For this review, take the finished solid that the model builds, in its own axes (mm). Round coordinates to 2 decimals unless told otherwise and drop trailing zeros. Order: outer loops, then holes, each group sorted by start corner. A loop starts at its lowest first (then second) coordinate and runs counter-clockwise, first axis right, second up.
```python
from build123d import *

# Parameters (mm, degrees)
F0_W     = 260.35
F0_H     = 25
F1_DEPTH = 7
F2_R     = 3.302
F3_DEPTH = 7
F4_W     = 30
F4_H     = 7
F5_DEPTH = 7


with BuildPart() as f1:
    # F0 (on Top) → F1 (new body)
    with BuildSketch(Plane.XY):
        Rectangle(F0_W, F0_H)
    extrude(amount=F1_DEPTH)

    # F2 (on face) → F3 (cut, through all)
    with BuildSketch(Plane.XY.offset(7)):
        with Locations((-120.175, 0)):
            Circle(F2_R)
        Circle(F2_R)
        with Locations((120.175, 0)):
            Circle(F2_R)
    extrude(amount=-F3_DEPTH, mode=Mode.SUBTRACT)

    # F4 (on face) → F5 (join)
    with BuildSketch(Plane(origin=(0, 12.5, 0), x_dir=(-1, 0, 0), z_dir=(0, 1, 0))):
        with Locations((100.175, 3.5)):
            Rectangle(F4_W, F4_H)
        with Locations((50.175, 3.5)):
            Rectangle(F4_W, F4_H)
        with Locations((-50.175, 3.5)):
            Rectangle(F4_W, F4_H)
        with Locations((-100.175, 3.5)):
            Rectangle(F4_W, F4_H)
    extrude(amount=F5_DEPTH)


solid = f1.part
```
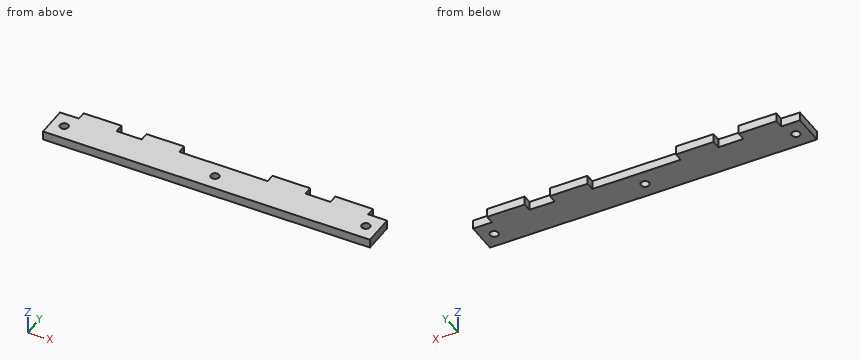
Q1. Take a section at B-B, the plane x = 0. State the section outline as (y, z) points.
Q2. Clearance check with flat-ended pins moving along their axes: pin 1 (3.5 mm diameter, centred on y = 16.5, z = 2.5, fed in from +X) (3 decimals); pin 2 (2 mm diameter, centred on x = -76.5, z = 2.5, fed in from +Y); pin 3 (2 mm diameter, centred on y = 14.5, z = 4.5, fed in from -X) (3 decimals). State where each tip first meets the part, or that it passes through.
Q3. Take a section at D-D, the plane y = 0. State the section outline as (x, z) points (3 decimals), plus the area to 3 significant figures.
Q4. Take a section at A-A, the plane y = 17. State the section outline as (x, z) points (3 decimals).
Q5. Wall thickness on line 1 (X direction, y = 13, z = 4.25) (3 decimals); line 2 (X direction, y = -1, z = 4) (3 decimals); line 3 (Y direction, x = -84, z = 4.5): over which ranges is each line inside the solid? List them lowest first.
Q6. Take a section at C-C, the plane z = 1.25. State the section outline as (x, y) points (3 decimals).
Working result:
1. outline: (-12.5, 0) - (-3.3, 0) - (-3.3, 7) - (-12.5, 7) - close; (3.3, 0) - (12.5, 0) - (12.5, 7) - (3.3, 7) - close
2. pin 1: stops at x = 115.175
2. pin 2: stops at y = 12.5
2. pin 3: stops at x = -115.175
3. outline: (-130.175, 0) - (-123.477, 0) - (-123.477, 7) - (-130.175, 7) - close; (-116.873, 0) - (-3.302, 0) - (-3.302, 7) - (-116.873, 7) - close; (3.302, 0) - (116.873, 0) - (116.873, 7) - (3.302, 7) - close; (123.477, 0) - (130.175, 0) - (130.175, 7) - (123.477, 7) - close
3. area: 1,680 mm2
4. outline: (-115.175, 0) - (-85.175, 0) - (-85.175, 7) - (-115.175, 7) - close; (-65.175, 0) - (-35.175, 0) - (-35.175, 7) - (-65.175, 7) - close; (35.175, 0) - (65.175, 0) - (65.175, 7) - (35.175, 7) - close; (85.175, 0) - (115.175, 0) - (115.175, 7) - (85.175, 7) - close
5. line 1: x = -115.175 to -85.175, -65.175 to -35.175, 35.175 to 65.175, 85.175 to 115.175
5. line 2: x = -130.175 to -123.322, -117.028 to -3.147, 3.147 to 117.028, 123.322 to 130.175
5. line 3: y = -12.5 to 12.5
6. outline: (-130.175, -12.5) - (130.175, -12.5) - (130.175, 12.5) - (115.175, 12.5) - (115.175, 19.5) - (85.175, 19.5) - (85.175, 12.5) - (65.175, 12.5) - (65.175, 19.5) - (35.175, 19.5) - (35.175, 12.5) - (-35.175, 12.5) - (-35.175, 19.5) - (-65.175, 19.5) - (-65.175, 12.5) - (-85.175, 12.5) - (-85.175, 19.5) - (-115.175, 19.5) - (-115.175, 12.5) - (-130.175, 12.5) - close; hole circle Ø6.604 at (-120.175, 0); hole circle Ø6.604 at (0, 0); hole circle Ø6.604 at (120.175, 0)
